from build123d import *

# Parameters (mm, degrees)
SKETCH1_W           = 70
SKETCH1_H           = 34
SKETCH1_R           = 2
BOSS_EXTRUDE1_DEPTH = 15
SKETCH6_W           = 70
SKETCH6_H           = 15
BOSS_EXTRUDE2_DEPTH = 5
SKETCH3_R           = 2
CUT_EXTRUDE2_DEPTH  = 15
SKETCH8_W           = 6
SKETCH8_H           = 5
CUT_EXTRUDE3_DEPTH  = 15
SKETCH9_W           = 12
SKETCH9_H           = 6
CUT_EXTRUDE4_DEPTH  = 15
SKETCH10_W          = 16
SKETCH10_H          = 10
CUT_EXTRUDE5_DEPTH  = 17
SKETCH12_R          = 1.5
CUT_EXTRUDE6_DEPTH  = 41
SKETCH13_W          = 27.5
SKETCH13_H          = 6
CUT_EXTRUDE7_DEPTH  = 20
SKETCH14_W          = 13.5
SKETCH14_H          = 2.67
SKETCH14_W_2        = 29
CUT_EXTRUDE8_DEPTH  = 17
FILLET2_R           = 4
SKETCH16_W          = 5.5
SKETCH16_H          = 3.33
CUT_EXTRUDE10_DEPTH = 18
FILLET4_R           = 4
FILLET5_R           = 4
SKETCH17_R          = 2.85
CUT_EXTRUDE11_DEPTH = 3
SKETCH18_R          = 2.8
CUT_EXTRUDE12_DEPTH = 3
CHAMFER1_SIZE       = 2
CHAMFER2_SIZE       = 2


# Some blends are built 0.0001 mm under size
with BuildPart() as part:
    # Sketch1 → Boss-Extrude1 (new body)
    with BuildSketch(Plane(origin=(0, 0, 0), x_dir=(1, 0, 0), z_dir=(0, 1, 0))):
        with Locations((-35, 17)):
            Rectangle(SKETCH1_W, SKETCH1_H)
        with Locations(Location((-35.1, 24, 0), (0, 0, 270))):
            Circle(SKETCH1_R, mode=Mode.SUBTRACT)
        with Locations(Location((-35.1, 5, 0), (0, 0, 270))):
            Circle(SKETCH1_R, mode=Mode.SUBTRACT)
    extrude(amount=BOSS_EXTRUDE1_DEPTH)

    # Sketch6 → Boss-Extrude2 (add)
    with BuildSketch(Plane.XY):
        with Locations((-35, 7.5)):
            Rectangle(SKETCH6_W, SKETCH6_H)
    extrude(amount=BOSS_EXTRUDE2_DEPTH)

    # Sketch3 → Cut-Extrude2 (cut)
    with BuildSketch(Plane(origin=(0, 15, 0), x_dir=(1, 0, 0), z_dir=(0, 1, 0))):
        with Locations(Location((-4, 1.67, 0), (0, 0, 270))):
            Circle(SKETCH3_R)
        with Locations(Location((-60.5, 1.67, 0), (0, 0, 270))):
            Circle(SKETCH3_R)
    extrude(amount=-CUT_EXTRUDE2_DEPTH, mode=Mode.SUBTRACT)

    # Sketch8 → Cut-Extrude3 (cut)
    with BuildSketch(Plane(origin=(0, 15, 0), x_dir=(1, 0, 0), z_dir=(0, 1, 0))):
        with Locations((-16.5, -2.5)):
            Rectangle(SKETCH8_W, SKETCH8_H)
    extrude(amount=-CUT_EXTRUDE3_DEPTH, mode=Mode.SUBTRACT)

    # Sketch9 → Cut-Extrude4 (cut)
    with BuildSketch(Plane(origin=(0, 15, 0), x_dir=(1, 0, 0), z_dir=(0, 1, 0))):
        with Locations((-35, -2)):
            Rectangle(SKETCH9_W, SKETCH9_H)
    extrude(amount=-CUT_EXTRUDE4_DEPTH, mode=Mode.SUBTRACT)

    # Sketch10 → Cut-Extrude5 (cut)
    with BuildSketch(Plane.XZ):
        with Locations((-8, -29)):
            Rectangle(SKETCH10_W, SKETCH10_H)
        with Locations((-62, -29)):
            Rectangle(SKETCH10_W, SKETCH10_H)
    extrude(amount=-CUT_EXTRUDE5_DEPTH, mode=Mode.SUBTRACT)

    # Sketch12 → Cut-Extrude6 (cut)
    with BuildSketch(Plane.XY.offset(5)):
        with Locations((-45, 7.5)):
            Circle(SKETCH12_R)
        with Locations((-25.499999999, 7.499999999)):
            Circle(SKETCH12_R)
    extrude(amount=-CUT_EXTRUDE6_DEPTH, mode=Mode.SUBTRACT)

    # Sketch13 → Cut-Extrude7 (cut)
    with BuildSketch(Plane(origin=(0, 15, 0), x_dir=(1, 0, 0), z_dir=(0, 1, 0))):
        with Locations((-27.25, -2)):
            Rectangle(SKETCH13_W, SKETCH13_H)
    extrude(amount=-CUT_EXTRUDE7_DEPTH, mode=Mode.SUBTRACT)

    # Sketch14 → Cut-Extrude8 (cut)
    with BuildSketch(Plane(origin=(0, 0, 0), x_dir=(-1, 0, 0), z_dir=(0, -1, 0))):
        with Locations((6.75, -3.665)):
            Rectangle(SKETCH14_W, SKETCH14_H)
        with Locations((55.5, -3.665)):
            Rectangle(SKETCH14_W_2, SKETCH14_H)
    extrude(amount=-CUT_EXTRUDE8_DEPTH, mode=Mode.SUBTRACT)

    # Fillet2
    fillet2_edges = [part.edges().sort_by_distance(p)[0] for p in [
        (0, 7.5, 2.33),
        (-70, 7.5, 2.33),
        (-70, 7.5, -24),
        (0, 7.5, -24),
    ]]
    fillet(fillet2_edges, radius=FILLET2_R)

    # Sketch16 → Cut-Extrude10 (cut)
    with BuildSketch(Plane.XZ):
        with Locations((-10.75, 0.665)):
            Rectangle(SKETCH16_W, SKETCH16_H)
    extrude(amount=-CUT_EXTRUDE10_DEPTH, mode=Mode.SUBTRACT)

    # Fillet4
    # the kernel refuses this fillet: 4 mm, written as the material it adds along each edge
    with BuildSketch(Plane(origin=(-16, 0, -24), x_dir=(1, 0, 0), z_dir=(0, 1, 0)), Plane(origin=(-54, 0, -24), x_dir=(0, 0, -1), z_dir=(0, 1, 0))) as fillet4_piece_1:
        with BuildLine():
            CenterArc((FILLET4_R, FILLET4_R), FILLET4_R, 180, 90)
            Line((0, FILLET4_R), (-FILLET4_R * 0.02, FILLET4_R))
            Line((-FILLET4_R * 0.02, FILLET4_R), (-FILLET4_R * 0.02, -FILLET4_R * 0.02))
            Line((-FILLET4_R * 0.02, -FILLET4_R * 0.02), (FILLET4_R, -FILLET4_R * 0.02))
            Line((FILLET4_R, -FILLET4_R * 0.02), (FILLET4_R, 0))
        make_face()
    extrude(amount=15)
    with BuildSketch(Plane(origin=(-41, 15, -1), x_dir=(0, 0, 1), z_dir=(0, -1, 0))) as fillet4_piece_2:
        with BuildLine():
            CenterArc((4, -3.943488304), FILLET4_R, 99.642495459, 80.357504541)
            Line((0, -3.943488304), (-0.08, -3.943488304))
            Line((-0.08, -3.943488304), (-0.08, 0))
            Line((-0.08, 0), (0, 0.08))
            ThreePointArc((0, 0.08), (1.665, 0.08), (3.3166, 0.078869766))
            Line((3.3166, 0.078869766), (3.33, 0))
        make_face()
    extrude(amount=15)
    with BuildSketch(Plane(origin=(-8, 0, -1), x_dir=(-1.0, 0, -8.691057696161095e-11), z_dir=(0, 1, 0))) as fillet4_piece_3:
        with BuildLine():
            CenterArc((3.943488303, 4), FILLET4_R, 189.642495464, 80.357504541)
            Line((0, 3.33), (-0.078869766, 3.3166))
            ThreePointArc((-0.078869766, 3.3166), (-0.08, 1.665), (-0.08, 0))
            Line((-0.08, 0), (0, -0.08))
            Line((0, -0.08), (3.943488304, -0.08))
            Line((3.943488304, -0.08), (3.943488304, 0))
        make_face()
    extrude(amount=15)

    # Fillet5
    fillet5_edges = [part.edges().sort_by_distance(p)[0] for p in [
        (-41, 7.5, 2.33),
        (-8, 7.5, 2.33),
    ]]
    fillet(fillet5_edges, radius=FILLET5_R)

    # Sketch17 → Cut-Extrude11 (cut)
    with BuildSketch(Plane.XY.offset(-1)):
        with Locations((-25.499999999, 7.499999999)):
            Circle(SKETCH17_R)
    extrude(amount=-CUT_EXTRUDE11_DEPTH, mode=Mode.SUBTRACT)

    # Sketch18 → Cut-Extrude12 (cut)
    with BuildSketch(Plane.XY.offset(2.33)):
        with Locations((-45, 7.5)):
            Circle(SKETCH18_R)
    extrude(amount=-CUT_EXTRUDE12_DEPTH, mode=Mode.SUBTRACT)

    # Chamfer1
    chamfer1_edges = [part.edges().sort_by_distance(p)[0] for p in [
        (-35.1, 0, -26),
    ]]
    chamfer(chamfer1_edges, length=CHAMFER1_SIZE)

    # Chamfer2
    chamfer2_edges = [part.edges().sort_by_distance(p)[0] for p in [
        (-35.1, 0, -7),
    ]]
    chamfer(chamfer2_edges, length=CHAMFER2_SIZE - 0.0001)  # a hair under: the kernel refuses the full size


solid = part.part
CAD build for the part. Positions are in the model's coordinates, mm. A direction names the side the tool comes from. Coordinates: 2 decimals unless noted, no trailing zeros. Write each loop counter-clockwise with the first axis right and the second up, starting at its lowest first coordinate (ties: lowest second). Pieces come first, ordered by that corner, then holes. Notation, with made-up numbers: (45.25, 64.25) - (79.25, 64.25) arc R8 ccw to (79.25, 71.25) - close; hole circle Ø11 at (31.5, 42.25). An arc over 180 degrees is marked (long way). Use a Markdown table: item, result. Add a question column.
Item 1: 3-axis set-ups, long thin cutter, end or side, ignore diameter. For faces 1 (the face through (-62, 7, -24)), 2 (the face through (-44, 6, -0.67)), 3 (the face through (-8, 7, -24)): which of +Z, -Z, +X, -X, +Y, -Y reach the whole face in a straight line?
Item 2: Band-saw the part on B-B, the plane x = -60.5. Give the cut face in (y, z).
Item 3: Drill centre lines: L1, parallel to Y at x = -25.5, z = -26.5; L2, parallel to Z at x = -16.5, y = 12.5; L3, parallel to X at y = 5.5, z = -29.5. Where is each one in solid material? Low to high. Write a range as from..to.
Item 4: Band-saw the part on C-C, the plane y = 4. Give the cut face in (x, z) (3 decimals).
Item 5: Band-saw the part on A-A, the plane z = -5. Give the cut face in (x, y), and give its area (3 significant figures).
Item 6: Band-saw the part on D-D, the plane x = -35.1. Give the number of separate pieces and of enclosed holes in the cut face, and give its area (3 significant figures).
Item 7: Flat gauge pins, fed straight in: pin 1 (6.5 mm diameter, centred on x = -26.5, y = 7, fed in from +Z); pin 2 (4.5 mm diameter, centred on x = -35.1, z = -5, fed in from -Y); pin 3 (6.5 mm diameter, centred on y = 10, z = -31, fed in from -X). Where does each tip first touch, or does it go through?
Item 8: Mould opens along Z. For faces 4 (the face through (-70, 7, -11)), 5 (the face through (-24, 6, -4)), 6 (the face through (-68.859, 7.605, -22.797)), 7 (the face through (-5.217, 7.605, -3.257)) say: pulls with the +Z half, pulls with the -Z half, needs draft (parallel to the pull), parting line crosses it, or undercut.
Numbers:
| question | item | result |
|---|---|---|
| 1 | face 1 | -Z, -X, +Y, -Y |
| 1 | face 2 | +Z |
| 1 | face 3 | -Z, +X, +Y, -Y |
| 2 | outline | (0, -24) - (15, -24) - (15, -3.67) - (0, -3.67) - close; (0, 0.33) - (15, 0.33) - (15, 2.33) - (0, 2.33) - close |
| 3 | L1 | 0..6, 9..15 |
| 3 | L2 | -34..-1 |
| 3 | L3 | -54..-16 |
| 4 | outline | (-70, -20) arc R4 ccw to (-66, -24) - (-58, -24) arc R4 cw to (-54, -28) - (-54, -34) - (-16, -34) - (-16, -28) arc R4 cw to (-12, -24) - (-4, -24) arc R4 ccw to (0, -20) - (0, -1.67) arc R4 ccw to (-4, 2.33) - (-5.448, 2.33) arc R4 ccw to (-8.696, 0.665) arc R4 cw to (-11.943, -1) - (-37.057, -1) arc R4 cw to (-40.304, 0.665) arc R4 ccw to (-43.552, 2.33) - (-66, 2.33) arc R4 ccw to (-70, -1.67) - close; hole circle Ø4 at (-60.5, -1.67); hole circle Ø4 at (-35.1, -24); hole circle Ø4 at (-35.1, -5); hole circle Ø4 at (-4, -1.67) |
| 5 | outline | (-70, 0) - (-39.1, 0) - (-37.1, 2) - (-37.1, 15) - (-70, 15) - close; (-33.1, 2) - (-31.1, 0) - (0, 0) - (0, 15) - (-33.1, 15) - close; hole circle Ø3 at (-45, 7.5); hole circle Ø3 at (-25.5, 7.5) |
| 5 | area | 972 mm2 |
| 6 | separate pieces | 3 |
| 6 | enclosed holes | 0 |
| 6 | area | 367 mm2 |
| 7 | pin 1 | z = -1 |
| 7 | pin 2 | y = 1.75 |
| 7 | pin 3 | x = -54.01 |
| 8 | face 4 | needs draft |
| 8 | face 5 | pulls with the +Z half |
| 8 | face 6 | pulls with the -Z half |
| 8 | face 7 | undercut |
